Build history of the part. All positions in model axes, mm. Face numbers are marked on the shaded views. A direction names the side the tool comes from. Round coordinates to 2 decimals unless told otherwise and drop trailing zeros. Write each loop counter-clockwise with the first axis right and the second up, starting at its lowest first coordinate (ties: lowest second). Pieces come first, ordered by that corner, then holes. Notation, with made-up numbers: M -14,-28.75 L 43,-28.75 A23 cw 43,10.25 Z; hole C 57,-10.5 d2. An arc over 180 degrees is marked long. Use a Markdown table: item, result.
from build123d import *

# Parameters (mm, degrees)
F1_DEPTH = 10
F3_DEPTH = 25
F4_SIZE  = 2
F6_D     = 3.3
F6_DEPTH = 10
F6_TIP   = 0.9914200214
F8_D     = 3.3
F8_DEPTH = 10
F8_TIP   = 0.9914200214


with BuildPart() as f1:
    # F0 (on Front) → F1 (new body, symmetric)
    with BuildSketch(Plane.XZ):
        with BuildLine():
            Line((7.5, -35), (37.5, -35))
            Line((37.5, -35), (37.5, 35))
            Line((37.5, 35), (10, 35))
            Line((10, 35), (-10, 35))
            Line((-10, 35), (-37.5, 35))
            Line((-37.5, 35), (-37.5, -35))
            Line((-37.5, -35), (-7.5, -35))
            Line((-7.5, -35), (-7.5, -17.867))
            ThreePointArc((-7.5, -17.867), (0, -10.367), (7.5, -17.867))
            Line((7.5, -17.867), (7.5, -35))
        make_face()
        with BuildLine():
            Line((-7.5, -35), (7.5, -35))
            Line((7.5, -35), (7.5, -17.867))
            ThreePointArc((7.5, -17.867), (0, -10.367), (-7.5, -17.867))
            Line((-7.5, -17.867), (-7.5, -35))
        make_face()
        Polygon((10, 35), (37.5, 35), (20.2677392039, 64.8471512281), (10, 64.8471512281), align=None)
        Polygon((-37.5, 35), (-10, 35), (-10, 64.8471512281), (-20.2677392039, 64.8471512281), align=None)
    extrude(amount=F1_DEPTH, both=True)

    # F2 (on Front) → F3 (cut, symmetric)
    with BuildSketch(Plane.XZ):
        with BuildLine():
            Line((-7.5, -17.867), (-7.5, -35))
            Line((-7.5, -35), (7.5, -35))
            Line((7.5, -35), (7.5, -17.867))
            ThreePointArc((7.5, -17.867), (0, -10.367), (-7.5, -17.867))
        make_face()
    extrude(amount=F3_DEPTH, both=True, mode=Mode.SUBTRACT)

    # F4
    f4_edges = [f1.edges().sort_by_distance(p)[0] for p in [
        (37.5, -10, 0),
        (28.88387, -10, 49.923576),
        (22.5, -10, -35),
        (-22.5, -10, -35),
        (-37.5, -10, 0),
        (-28.88387, -10, 49.923576),
        (-15.13387, -10, 64.847151),
        (15.13387, -10, 64.847151),
    ]]
    chamfer(f4_edges, length=F4_SIZE)

    # F6
    with Locations(Plane.XZ.offset(10)):
        with Locations((0, -5.952)):
            Hole(F6_D / 2, depth=F6_DEPTH)
            with Locations((0, 0, -(F6_DEPTH + F6_TIP / 2))):  # 118° drill point
                Cone(0, F6_D / 2, F6_TIP, mode=Mode.SUBTRACT)

    # F8
    with Locations(Plane.XY.offset(35)):
        with Locations((0, 0)):
            Hole(F8_D / 2, depth=F8_DEPTH)
            with Locations((0, 0, -(F8_DEPTH + F8_TIP / 2))):  # 118° drill point
                Cone(0, F8_D / 2, F8_TIP, mode=Mode.SUBTRACT)


solid = f1.part
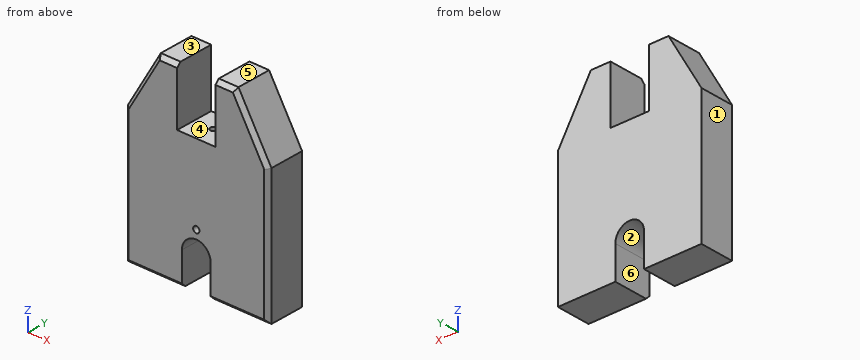
Q1. Cut at A-A on y = -4.5. Give the cut face in (x, z), and give its area (3 significant figures).
Response values:
| item | result |
|---|---|
| outline | M -37.5,-35 L -7.5,-35 L -7.5,-17.87 A7.5 cw 7.5,-17.87 L 7.5,-35 L 37.5,-35 L 37.5,35 L 20.27,64.85 L 10,64.85 L 10,35 L -10,35 L -10,64.85 L -20.27,64.85 L -37.5,35 Z; hole C 0,-5.95 d3.3 |
| area | 6,020 mm2 |
Q2. Drill centre lines: L1, parallel to Y at x = 0, z = 32.5; L2, parallel to Z at x = 0, y = -2; L3, parallel to X at y = -2.5, z = 38.5. Where is each one in solid material? Low to high.
Response values:
| item | result |
|---|---|
| L1 | y = -10 to -1.65, 1.65 to 10 |
| L2 | z = -10.37 to -7.6, -4.3 to 35 |
| L3 | x = -35.48 to -10, 10 to 35.48 |
Q3. Drop flat-ended pins along their axis: P1, Ø6, axis at y = 1, z = 47, coming from the -X side; P2, Ø2, axis at x = 0, y = 0, coming from the -Z side; P3, Ø6, axis at x = -4.5, y = -4, coming from the +Z side. Give the stop position or say it passes through.
Response values:
| item | result |
|---|---|
| P1 | stops at x = -32.3 |
| P2 | stops at z = -10.43 |
| P3 | stops at z = 35 |
Q4. Two-plate mould, pull along X, no slides. Class the marked faces 1, 2 and 3: +X half, -X half, draft (parallel to the pull), parting line (faces both ways), or undercut.
Response values:
| item | result |
|---|---|
| face 1 | -X half |
| face 2 | undercut |
| face 3 | draft |
Q5. Cut at B-B on z = 58.5. Give the cut face in (x, y).
Response values:
| item | result |
|---|---|
| outline | M -23.93,-8 L -21.62,-10 L -10,-10 L -10,10 L -23.93,10 Z; M 10,-10 L 21.62,-10 L 23.93,-8 L 23.93,10 L 10,10 Z |
Q6. Which spindle directions (+Z, -Z, +X, -X, +Y, -Y) get a long thin tool onto all of the face, cutting with end or side? Do the marked faces 4, 5 and 6. Say none if no direction does.
Response values:
| item | result |
|---|---|
| face 4 | +Z, +Y, -Y |
| face 5 | +Z, +X, -X, +Y, -Y |
| face 6 | -Z, +Y, -Y |
Q7. Cut at C-C on y = 5. Give the cut face in (x, z), and give its area (3 significant figures).
Response values:
| item | result |
|---|---|
| outline | M -37.5,-35 L -7.5,-35 L -7.5,-17.87 A7.5 cw 7.5,-17.87 L 7.5,-35 L 37.5,-35 L 37.5,35 L 20.27,64.85 L 10,64.85 L 10,35 L -10,35 L -10,64.85 L -20.27,64.85 L -37.5,35 Z |
| area | 6,030 mm2 |
